from build123d import *

# Parameters (mm, degrees)
SKETCH4_W           = 50.7492
SKETCH4_H           = 101.6
BOSS_EXTRUDE2_DEPTH = 50.8
CUT_EXTRUDE2_DEPTH  = 125.413348563
SKETCH7_W           = 33.8328
SKETCH7_H           = 33.8328
BOSS_EXTRUDE3_DEPTH = 0.5588
SKETCH8_R           = 16.9164
BOSS_EXTRUDE4_DEPTH = 50.8


with BuildPart() as part:
    # Sketch4 → Boss-Extrude2 (new body)
    with BuildSketch(Plane.XY):
        with Locations((-25.3746, 50.8)):
            Rectangle(SKETCH4_W, SKETCH4_H)
        with Locations((25.3746, 50.8)):
            Rectangle(SKETCH4_W, SKETCH4_H)
    extrude(amount=-BOSS_EXTRUDE2_DEPTH)

    # Sketch5 → Cut-Extrude2 (cut, through all)
    with BuildSketch(Plane.XY):
        Polygon((-6.3246, 101.6), (6.3246, 101.6), (6.3246, 63.5254), (31.70428, 63.5254), (31.70428, 25.4508), (-31.70428, 25.4508), (-31.70428, 63.5254), (-6.3246, 63.5254), align=None)
    extrude(amount=-CUT_EXTRUDE2_DEPTH, mode=Mode.SUBTRACT)

    # Sketch7 → Boss-Extrude3 (add)
    with BuildSketch(Plane(origin=(0, 0, -50.8), x_dir=(-1, 0, 0), z_dir=(0, 0, -1))):
        with Locations((-0.043435031, -16.9164)):
            Rectangle(SKETCH7_W, SKETCH7_H)
    extrude(amount=-BOSS_EXTRUDE3_DEPTH)

    # Sketch8 → Boss-Extrude4 (add)
    with BuildSketch(Plane(origin=(0, 0, -50.8), x_dir=(-1, 0, 0), z_dir=(0, 0, -1))):
        with Locations((-0.043435031, -33.8328)):
            Circle(SKETCH8_R)
    extrude(amount=-BOSS_EXTRUDE4_DEPTH)


solid = part.part
Verification items for the finished model (mm, model axes). A direction names the side the tool comes from. Give positions to 0.01 mm unless a question says otherwise; leave off trailing zeros. Order: outer loops, then holes, each group sorted by start corner. A loop starts at its lowest first (then second) coordinate and runs counter-clockwise, first axis right, second up. Notation, with made-up numbers: (17.25, -31.5) -> (42.25, -31.5) arc R26 cw to (42.25, -17.5) -> close; hole circle Ø7 at (-30, -5). An arc over 180 degrees is marked (long way). Answer as CSV lines item,"result".
Q1. Release check for a two-part mould opening along Y. For faces 1 (the flat face through (0, -9, -50.241)), 2 (the flat face through (29, 101.6, -25)), 3 (the flat face through (-50.749, 50, -25)) record: +Y half, -Y half, draft (parallel to the pull), parting line (faces both ways), or undercut.
Solutions:
face 1,"undercut"
face 2,"+Y half"
face 3,"draft"
Q2. Depth check by flat-ended pin: pin 1 (10 mm diameter, centred on x = 5.5, y = -8.5, fed in from +Z); pin 2 (20.5 mm diameter, centred on x = -15, z = -30, fed in from -Y); pin 3 (3 mm diameter, centred on x = -28, z = -45.5, fed in from -Y). Enter the tip coordinate at first touch or a pass-through.
Solutions:
pin 1,"stops at z = -50.24"
pin 2,"stops at y = -50.06"
pin 3,"stops at y = 0"
Q3. Access from +Z, -Z, +X, -X, +Y, -Y to the whole of each face (thin tool, end or side, straight path). Record for faces 4 (the flat face through (6.325, 83, -25)), 5 (the flat face through (19, 63.525, -25)), 6 (the cylindrical face through (2.25, -17.06, -25.76)), 7 (the flat face through (-28, 101.6, -25)), 8 (the flat face through (0, -34, 0)).
Solutions:
face 4,"+Z, -Z, +Y"
face 5,"+Z, -Z"
face 6,"+Z"
face 7,"+Z, -Z, +X, -X, +Y"
face 8,"+Z, +X, -X, +Y, -Y"
Q4. Sectioned sample at C-C on y = 49. Record the cut outline in (x, z).
Solutions:
outline,"(-50.75, -50.8) -> (-31.7, -50.8) -> (-31.7, 0) -> (-50.75, 0) -> close; (31.7, -50.8) -> (50.75, -50.8) -> (50.75, 0) -> (31.7, 0) -> close"
Q5. Sectioned sample at B-B on x = -12.5. Record the cut outline in (y, z), plus the area to 3 significant figures.
Solutions:
outline,"(-45.18, -50.8) -> (25.45, -50.8) -> (25.45, 0) -> (0, 0) -> (0, -50.24) -> (-22.48, -50.24) -> (-22.48, 0) -> (-45.18, 0) -> close; (63.53, -50.8) -> (101.6, -50.8) -> (101.6, 0) -> (63.53, 0) -> close"
area,"4,390 mm²"
Q6. Scan lines: probe 1 along Y at (x, z) = (-1, -42); probe 2 along Y at (x, z) = (12.5, -33); probe 3 along Y at (x, z) = (-26, -8). Record each from-to range of solid material in increasing order.
Solutions:
probe 1,"y = -50.72 to -16.95, 0 to 25.45"
probe 2,"y = -45.28 to -22.39, 0 to 25.45, 63.53 to 101.6"
probe 3,"y = 0 to 25.45, 63.53 to 101.6"
Q7. Sectioned sample at D-D on x = -25. Record the cut outline in (y, z), plus the area to 3 significant figures.
Solutions:
outline,"(0, -50.8) -> (25.45, -50.8) -> (25.45, 0) -> (0, 0) -> close; (63.53, -50.8) -> (101.6, -50.8) -> (101.6, 0) -> (63.53, 0) -> close"
area,"3,230 mm²"
Q8. Sectioned sample at A-A on z = -8. Record the cut outline in (x, y).
Solutions:
outline,"(-50.75, 0) -> (50.75, 0) -> (50.75, 101.6) -> (6.32, 101.6) -> (6.32, 63.53) -> (31.7, 63.53) -> (31.7, 25.45) -> (-31.7, 25.45) -> (-31.7, 63.53) -> (-6.32, 63.53) -> (-6.32, 101.6) -> (-50.75, 101.6) -> close; circle Ø33.83 at (0.04, -33.83)"
